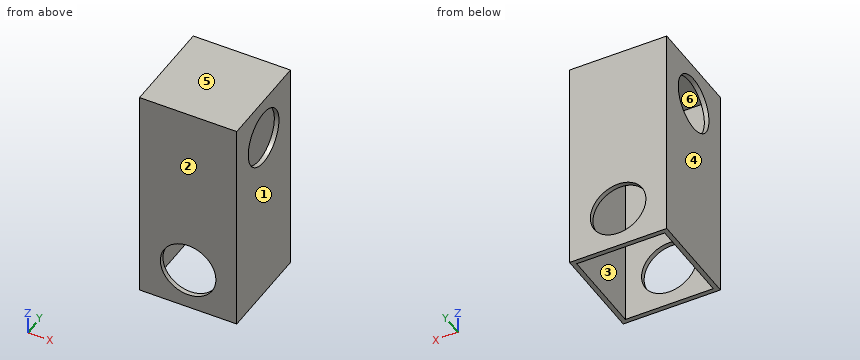
```python
from build123d import *

# Parameters (mm, degrees)
F0_W     = 42
F0_H     = 94
F1_DEPTH = 21
F3_T     = -2
F2_R     = 12
F4_DEPTH = 38.1
F5_R     = 12
F6_DEPTH = 38.1


with BuildPart() as f1:
    # F0 (on Front) → F1 (new body, symmetric)
    with BuildSketch(Plane.XZ):
        Rectangle(F0_W, F0_H)
    extrude(amount=F1_DEPTH, both=True)

    # F3
    f3_openings = [f1.faces().sort_by_distance(p)[0] for p in [
        (0, 0, -47),
    ]]
    offset(amount=F3_T, openings=f3_openings)

    # F2 (on Front) → F4 (cut, symmetric)
    with BuildSketch(Plane.XZ):
        with Locations((0, -29)):
            Circle(F2_R)
    extrude(amount=F4_DEPTH, both=True, mode=Mode.SUBTRACT)

    # F5 (on Right) → F6 (cut, symmetric)
    with BuildSketch(Plane.YZ):
        with Locations((0, 29)):
            Circle(F5_R)
    extrude(amount=F6_DEPTH, both=True, mode=Mode.SUBTRACT)


solid = f1.part
```
Geometry check sheet. Reference: the model listing, model coordinates, mm. Face numbers are marked on the shaded views. A direction names the side the tool comes from. Give positions to 0.01 mm unless a question says otherwise; leave off trailing zeros. Loops run counter-clockwise (first coordinate to the right, second up) from the corner with the lowest first, then second, coordinate; pieces in that order, holes last. Notation, with made-up numbers: M -3.75,72 L 7.25,72 A22 ccw 7.25,95 Z; hole C 59.5,-40 d1. An arc over 180 degrees is marked long. Write item = value, one per line. Start each with the question number.
1. Section check D-D, the plane z = -9. Enter the section's corners in (x, y), plus the area to 3 significant figures.
2. Go/stop test with flat-tipped pins: P1, Ø19, axis at y = 0, z = 29, coming from the +X side; P2, Ø11.5, axis at x = 7, y = 8.5, coming from the -Z side. Record where each tip stops, or that it passes through.
3. Section check C-C, the plane x = -13. Enter the section's corners in (y, z), plus the area to 3 significant figures.
4. Draft check along X on the marked faces 1, 2, 3 and 4. Enter one of: +X half, -X half, draft (parallel to the pull), parting line (faces both ways), or undercut.
5. Section check B-B, the plane y = 0. Enter the section's corners in (x, z).
6. Tool access check on the marked faces 5 and 6. Record the directions out of +Z, -Z, +X, -X, +Y, -Y that give a thin tool (end or side, any length) a straight path to the whole face; none if there is none.
7. Thickness scan on probe 1 along Y at (x, z) = (-18, 25); probe 2 along Z at (x, y) = (0, -19.8). Record the ranges inside material, lowest first.
8. Section check A-A, the plane z = 29. Enter the section's corners in (x, y), plus the area to 3 significant figures.
Values follow:
q1.outline = M -21,-21 L 21,-21 L 21,21 L -21,21 Z; hole M -19,-19 L 19,-19 L 19,19 L -19,19 Z
q1.area = 320 mm^2
q2.P1 = through
q2.P2 = 45
q3.outline = M -21,-47 L -19,-47 L -19,45 L 19,45 L 19,-47 L 21,-47 L 21,47 L -21,47 Z
q3.area = 452 mm^2
q4.face_1 = +X half
q4.face_2 = draft
q4.face_3 = undercut
q4.face_4 = -X half
q5.outline = M -21,-47 L -19,-47 L -19,17 L -21,17 Z; M -21,41 L -19,41 L -19,45 L 19,45 L 19,41 L 21,41 L 21,47 L -21,47 Z; M 19,-47 L 21,-47 L 21,17 L 19,17 Z
q6.face_5 = +Z, +X, -X, +Y, -Y
q6.face_6 = -Z
q7.probe_1 = -21 to -19, 19 to 21
q7.probe_2 = -47 to -41, -17 to 47
q8.outline = M -21,-21 L 21,-21 L 21,-12 L 19,-12 L 19,-19 L -19,-19 L -19,-12 L -21,-12 Z; M -21,12 L -19,12 L -19,19 L 19,19 L 19,12 L 21,12 L 21,21 L -21,21 Z
q8.area = 224 mm^2
